The listing builds one solid part. Answer for the finished solid, in the listing's coordinates (mm). A direction names the side the tool comes from. Give positions to 0.01 mm unless a question says otherwise; leave off trailing zeros. Loops run counter-clockwise (first coordinate to the right, second up) from the corner with the lowest first, then second, coordinate; pieces in that order, holes last.
Item 1: Section B-B, the plane y = 4 is taken. Give the vertices of the cut face in (x, z).
Item 2: Consider line 1 along X through (y, z) = (22, -2.2); line 2 along Y through (x, z) = (-9.5, -1.7); line 3 along Z through (x, y) = (20, -6). Determine where each line is inside the solid, lowest interval first.
Item 3: Section C-C, the plane x = -20 is taken. Give the vertices of the cut face in (y, z).
Item 4: This flat-tipped pin is pushed along its axis until it touches: pin 1 Ø1.5 at (x, y) = (15.5, -12.5) entering from +Z. Where does it stop, or does it pass through?
Item 5: Section A-A, the plane z = -2.9 is taken. Give the vertices of the cut face in (x, y).
Item 6: The mould has two halves that part along X. Classify faces 1 (the face through (36, -1, -2)), 2 (the face through (38, 1, -3)), 3 (the face through (-38, 1, -3)): pulls with the +X half, pulls with the -X half, needs draft (parallel to the pull), parting line crosses it, or undercut.
Item 7: A tool of negligible diameter and unlimited length cuts with its end or side. For faces 4 (the face through (-1, -1, -6)), 5 (the face through (-1, 1, -4)), from which of +Z, -Z, +X, -X, +Y, -Y can it reach the whole face along a straight path? Write none if from no direction.
from build123d import *

# Parameters (mm, degrees)
SKETCH005_W     = 76
SKETCH005_H     = 81
PAD001_DEPTH    = 6
SKETCH006_W     = 72
SKETCH006_H     = 77
POCKET004_DEPTH = 4
CHAMFER002_SIZE = 1


with BuildPart() as part:
    # Sketch005 (on Face1 of CopyChamfer001) → Pad001 (new body)
    with BuildSketch(Plane(origin=(0, 0, 0), x_dir=(1, 0, 0), z_dir=(0, 0, -1))):
        Rectangle(SKETCH005_W, SKETCH005_H)
    extrude(amount=PAD001_DEPTH)

    # Sketch006 (on Face5 of Pad001) → Pocket004 (cut)
    with BuildSketch(Plane.XY):
        Rectangle(SKETCH006_W, SKETCH006_H)
    extrude(amount=-POCKET004_DEPTH, mode=Mode.SUBTRACT)

    # Chamfer002
    chamfer002_edges = [part.edges().sort_by_distance(p)[0] for p in [
        (36, -38.5, -2),
        (-36, -38.5, -2),
        (-36, 38.5, -2),
        (36, 38.5, -2),
        (38, -40.5, -3),
        (-38, -40.5, -3),
        (38, 40.5, -3),
        (-38, 40.5, -3),
        (0, 40.5, 0),
        (-38, 0, 0),
        (0, -40.5, 0),
        (38, 0, 0),
    ]]
    chamfer(chamfer002_edges, length=CHAMFER002_SIZE)


solid = part.part
Worked answers:
1. outline: (-38, -6) - (38, -6) - (38, -1) - (37, 0) - (36, 0) - (36, -4) - (-36, -4) - (-36, 0) - (-37, 0) - (-38, -1) - close
2. line 1: x = -38 to -36, 36 to 38
2. line 2: y = -40.5 to -38.5, 38.5 to 40.5
2. line 3: z = -6 to -4
3. outline: (-40.5, -6) - (40.5, -6) - (40.5, -1) - (39.5, 0) - (38.5, 0) - (38.5, -4) - (-38.5, -4) - (-38.5, 0) - (-39.5, 0) - (-40.5, -1) - close
4. pin 1: stops at z = -4
5. outline: (-38, -39.5) - (-37, -40.5) - (37, -40.5) - (38, -39.5) - (38, 39.5) - (37, 40.5) - (-37, 40.5) - (-38, 39.5) - close; hole (-36, -37.5) - (-35, -38.5) - (35, -38.5) - (36, -37.5) - (36, 37.5) - (35, 38.5) - (-35, 38.5) - (-36, 37.5) - close
6. face 1: undercut
6. face 2: pulls with the +X half
6. face 3: pulls with the -X half
7. face 4: -Z, +X, -X, +Y, -Y
7. face 5: +Z
